Source: CAD feature listing. Evaluate the final solid. Frame: model axes, mm. Round coordinates to 2 decimals unless told otherwise and drop trailing zeros. Write each loop counter-clockwise with the first axis right and the second up, starting at its lowest first coordinate (ties: lowest second). Pieces come first, ordered by that corner, then holes. Notation, with made-up numbers: M 51.25,29.5 L 59.25,29.5 A30 cw 59.25,53.5 Z; hole C 29.25,-34.75 d4. An arc over 180 degrees is marked long. Answer in a Markdown table with one row per item. Add a question column.
Item 1: Material intervals for probe 1 along Y at (x, z) = (40.25, 14.5); probe 2 along Z at (x, y) = (38.25, 55); probe 3 along X at (y, z) = (50.75, 3.5), sorted ascending.
Item 2: Cut plane A-A on z = 22. Return loops of the section in (x, y).
Item 3: Contact query for flat-ended pins moving along their axis: pin 1 (6 mm diameter, centred on x = 44.5, z = 15, fed in from +Y); pin 2 (3 mm diameter, centred on x = 38, z = 13.5, fed in from -Y); pin 3 (8 mm diameter, centred on x = 44.5, y = 57.5, fed in from +Z). Output: stop coordinate, or through.
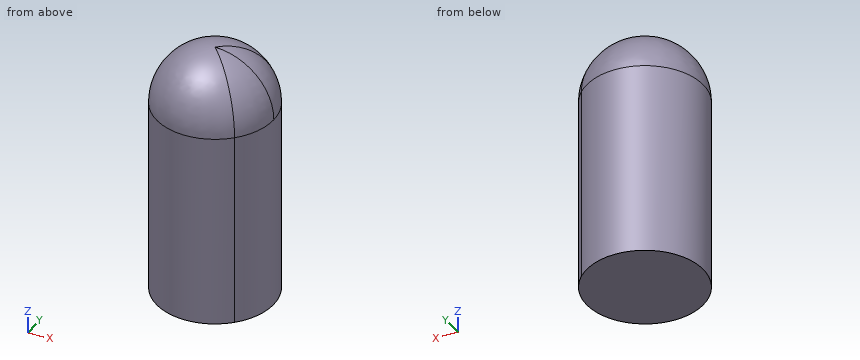
Autodesk Inventor part; units mm, degrees
ref_plane "YZ Plane" through (0, 0, 0) normal (1, 0, 0) x (0, 1, 0)
ref_plane "XZ Plane" through (0, 0, 0) normal (0, 1, 0) x (-1, 0, 0)
ref_plane "XY Plane" through (0, 0, 0) normal (0, 0, 1) x (1, 0, 0)
sketch "Sketch1" plane through (0, 0, 0) normal (0, 0, 1) x (1, 0, 0)
  arc A0 (45.3033, 58.3033) -> (45.3033, 47.6967) centre (40, 53) ccw
  circle A1 centre (40, 53) radius 7.5
  point P0 (0, 0)
extrude "Extrusion1" add sketch "Sketch1" along normal blind 32.5
fillet "Fillet1" radius 7.5 1 edges at (32.5, 53, 32.5)
properties part number "NotchPiston1"
Results below:
| question | item | result |
|---|---|---|
| 1 | probe 1 | 45.5 to 60.5 |
| 1 | probe 2 | 0 to 32.01 |
| 1 | probe 3 | 32.85 to 47.15 |
| 2 | outline | C 40,53 d15 |
| 3 | pin 1 | y = 60.35 |
| 3 | pin 2 | y = 45.52 |
| 3 | pin 3 | z = 32.12 |
